Geometry check sheet. Reference: drawing and pictorial views, mm from the part's lowest x, y, z. A direction names the side the tool comes from. Round coordinates to 2 decimals unless told otherwise and drop trailing zeros. Order: outer loops, then holes, each group sorted by start corner. A loop starts at its lowest first (then second) coordinate and runs counter-clockwise, first axis right, second up.
(1) Cross-section at A-A on x = 50. Enter the section's corners in (y, z).
(2) Thickness scan on L1, parallel to X at y = 1.2, z = 17.5; L2, parallel to Y at x = 50, z = 9; L3, parallel to X at y = 19.5, z = 5. Record the ranges inside material, lowest first.
(3) Cross-section at B-B on z = 17.5. Enter the section's corners in (x, y).
(4) Cross-section at D-D on x = 90. Enter the section's corners in (y, z).
(5) Draft check along X on the marked faces 4, 5 and 6. Enter one of: pulls with the +X half, pulls with the -X half, needs draft (parallel to the pull), parting line crosses it, or undercut.
(6) Cross-section at C-C on z = 11. Enter the section's corners in (x, y), and give its area (3 significant figures).
(7) Set-up check for the marked faces 1, 2 and 3: record each of +Z, -Z, +X, -X, +Y, -Y from which the full face is reachable in a straight line by a thin tool's end or side.
(8) Gauge pin test, flat ends, axial feed: P1, Ø1.5, axis at x = 63, z = 9, coming from the +Y side; P2, Ø6, axis at x = 90.5, z = 20, coming from the +Y side; P3, Ø8.5, axis at y = 25.5, z = 22.5, coming from the -X side; P4, Ø23.5, axis at x = 50, y = 43.8, coming from the +Z side. Record the tip position at first contact, or that the pin passes through.
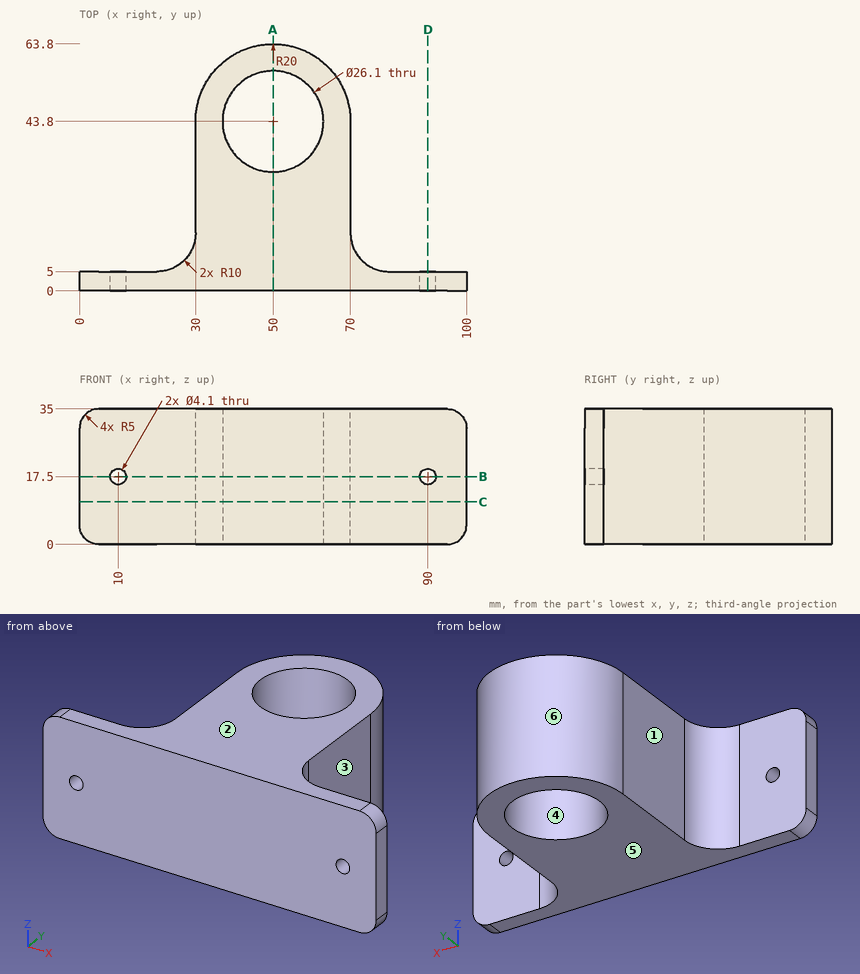
Found:
1. outline: (0, 0) - (30.75, 0) - (30.75, 35) - (0, 35) - close; (56.85, 0) - (63.8, 0) - (63.8, 35) - (56.85, 35) - close
2. L1: x = 0 to 7.95, 12.05 to 87.95, 92.05 to 100
2. L2: y = 0 to 30.75, 56.85 to 63.8
2. L3: x = 30 to 70
3. outline: (0, 0) - (7.95, 0) - (7.95, 5) - (0, 5) - close; (12.05, 0) - (87.95, 0) - (87.95, 5) - (80, 5) arc R10 cw to (70, 15) - (70, 43.8) arc R20 ccw to (30, 43.8) - (30, 15) arc R10 cw to (20, 5) - (12.05, 5) - close; (92.05, 0) - (100, 0) - (100, 5) - (92.05, 5) - close; hole circle Ø26.1 at (50, 43.8)
4. outline: (0, 0) - (5, 0) - (5, 15.45) - (0, 15.45) - close; (0, 19.55) - (5, 19.55) - (5, 35) - (0, 35) - close
5. face 4: undercut
5. face 5: needs draft
5. face 6: parting line crosses it
6. outline: (0, 0) - (100, 0) - (100, 5) - (80, 5) arc R10 cw to (70, 15) - (70, 43.8) arc R20 ccw to (30, 43.8) - (30, 15) arc R10 cw to (20, 5) - (0, 5) - close; hole circle Ø26.1 at (50, 43.8)
6. area: 2,190 mm2
7. face 1: +Z, -Z, -X, +Y
7. face 2: +Z, +X, -X, +Y, -Y
7. face 3: +Z, -Z, +X, +Y
8. P1: stops at y = 59.61
8. P2: stops at y = 5
8. P3: stops at x = 30
8. P4: passes through
